For this review, take the finished solid that the model builds, in its own axes (mm). A direction names the side the tool comes from. Coordinates: 2 decimals unless noted, no trailing zeros. Loops run counter-clockwise (first coordinate to the right, second up) from the corner with the lowest first, then second, coordinate; pieces in that order, holes last. Notation, with made-up numbers: M 44.25,59 L 86.25,59 A20 cw 86.25,63 Z; hole C -4,2.25 d11. An arc over 180 degrees is marked long. Write item = value, one per line.
Autodesk Fusion 360 part; units mm, degrees
sketch "Sketch1" plane through (0, 0, 0) normal (0, 1, 0) x (1, 0, 0)
  circle A0 centre (0, 0) radius 13
  circle A1 centre (0, 0) radius 21.25
  dimension "d1" = 26
  dimension "d2" = 42.5
extrude "Extrude1" add sketch "Sketch1" against normal blind 5 contours A0
extrude "Extrude2" add sketch "Sketch1" along normal blind 2.8 contours A0 | A1
sketch "Sketch2" plane through (0, 2.8, 0) normal (0, 1, 0) x (-1, 0, 0)
  circle A0 centre (0, 0) radius 21.25
  circle A1 centre (0, 0) radius 11
  dimension "d7" = 22
extrude "Extrude3" add sketch "Sketch2" along normal blind 13 contours A1
fillet "Fillet1" radius 4 1 edges at (10.2556, 2.8, 3.9778)
fillet "Fillet2" radius 10 1 edges at (10.2556, 15.8, -3.9778)
fillet "Fillet3" radius 2 1 edges at (-12.1203, 0, 4.701)
fillet "Fillet4" radius 2 1 edges at (-12.1203, -5, -4.701)
sketch "Sketch3" plane through (0, 2.8, 0) normal (0, 1, 0) x (-1, 0, 0)
  circle A0 centre (0, 0) radius 21.25
  circle A1 centre (0, 0) radius 15
  circle A2 centre (0, 0) radius 18.75
  circle A3 centre (0, 18.75) radius 1.6
  circle A4 centre (-16.238, -9.375) radius 1.6
  circle A5 centre (16.238, -9.375) radius 1.6
  dimension "d18" = 37.5
  dimension "d19" = 3.2
  dimension "d21" = 360
extrude "Extrude4" cut sketch "Sketch3" against normal blind 5 contours A2 A3 | A2 A3 | A2 A5 | A2 A5 | A2 A4 | A2 A4
equation "d18 = 42.500 mm - 5 mm"
Q1. Machinability: for faces 5 (the face through (4.4, 0, -14.5)), 6 (the face through (4.4, 2.8, -14.5)), 7 (the face through (-16.863, 1.38, -12.93)), which of the approach directions +Z, -Z, +X, -X, +Y, -Y give a long, thin tool a straight path to every point of the face, cutting with its end or side? Answer none if there is none.
Solved:
face_5 = -Y
face_6 = +Y
face_7 = +Y, -Y
Q2. For line 1 along Y through (x, z) = (-16.5, 5.5); line 2 along X through (y, z) = (1.35, 18.75); line 3 along X through (y, z) = (-3, 0.5), list the stretches that pass through material, from the lowest coordinate up.
Solved:
line_1 = 0 to 2.8
line_2 = -10 to -1.6, 1.6 to 10
line_3 = -12.99 to 12.99
Q3. Add section A-A (z = 18.75). Write out the cut boundary in (x, y), and give its area (3 significant figures).
Solved:
outline = M -10,0 L -1.6,0 L -1.6,2.8 L -10,2.8 Z; M 1.6,0 L 10,0 L 10,2.8 L 1.6,2.8 Z
area = 47.0 mm²
Q4. Add section B-B (z = -16.5). Write out the cut boundary in (x, y), and give its area (3 significant figures).
Solved:
outline = M -13.39,0 L 13.39,0 L 13.39,2.8 L -13.39,2.8 Z
area = 75.0 mm²
Q5. For pin 1 Ø3.5 at (x, z) = (-16.238, -9.375) entering from -Y; pin 2 Ø13 at (x, z) = (-7, -2.5) entering from +Y; pin 3 Ø3 at (x, z) = (16.238, -9.375) entering from -Y; pin 4 Ø3.5 at (x, z) = (0, 18.75) entering from +Y, all flat-tipped, find the tip position at first contact; note any pin that passes through.
Solved:
pin_1 = 0
pin_2 = 15.8
pin_3 = through
pin_4 = 2.8
Q6. Draft analysis for pull direction Z (two halves, no side actions). For faces 1 (the face through (0, 15.8, 0)), 2 (the face through (-16.976, 1.42, -10.794)), 3 (the face through (0.208, 1.42, 20.336)), 4 (the face through (-10.316, -2.493, 7.91)), state which applies: +Z half, -Z half, draft (parallel to the pull), parting line (faces both ways), or undercut.
Solved:
face_1 = draft
face_2 = undercut
face_3 = undercut
face_4 = parting line
